Check sheet for the modelled part. Datum: model origin and axes. Units: mm. A direction names the side the tool comes from. Give positions to 0.01 mm unless a question says otherwise; leave off trailing zeros. Write each loop counter-clockwise with the first axis right and the second up, starting at its lowest first coordinate (ties: lowest second). Pieces come first, ordered by that corner, then holes. Notation, with made-up numbers: M 12.5,16 L 45.5,16 A20 cw 45.5,50 Z; hole C 61.5,77 d3. An arc over 180 degrees is marked long. Write item = value, one per line. Start each with the question number.
1) Sectioned sample at C-C, the plane x = 1. Record the cut outline in (y, z).
2) Sectioned sample at A-A, the plane y = -17.25. Record the cut outline in (x, z) (3 decimals), then the cut area to 3 significant figures.
3) Draft check along X on faces 1 (the face through (12.7, -3, 5)), 2 (the face through (19.297, -13.993, 1.565)), 3 (the face through (16, -11, 3.175)). Enter one of: pulls with the +X half, pulls with the -X half, needs draft (parallel to the pull), parting line crosses it, or undercut.
4) Sectioned sample at B-B, the plane z = 1. Record the cut outline in (x, y) (3 decimals), then the cut area to 3 significant figures.
5) Sectioned sample at D-D, the plane x = 19.05. Record the cut outline in (y, z) (3 decimals).
6) Scan lines: L1, parallel to X at y = -16.5, z = 3; L2, parallel to X at y = -3.25, z = 5.5; L3, parallel to X at y = -3, z = 0.5. Record each from-to range of solid material in increasing order.
7) Set-up check for faces 4 (the face through (-12.7, -3, 5)), 5 (the face through (0, -12.7, 3)), 6 (the face through (-9.935, -11.591, 3.836)): record each of +Z, -Z, +X, -X, +Y, -Y from which the full face is reachable in a straight line by a thin tool's end or side.
8) Gauge pin test, flat ends, axial feed: pin 1 (2 mm diameter, centred on y = -7.5, z = 10, fed in from +X); pin 2 (3 mm diameter, centred on x = -6, y = -11, fed in from +Z); pin 3 (5 mm diameter, centred on x = 14.5, y = -8, fed in from +Z). Record the tip position at first contact, or that the pin passes through.
from build123d import *

# Parameters (mm, degrees)
BOSS_EXTRUDE1_DEPTH   = 12.7
BOSS_EXTRUDE2_DEPTH   = 3.175
FILLET1_R             = 6.35
F_6_CLEARANCE_HOLE1_D = 3.7973


with BuildPart() as part:
    # Sketch1 → Boss-Extrude1 (new body)
    with BuildSketch(Plane.XY):
        with BuildLine():
            Line((-12.7, 0), (12.7, 0))
            Line((12.7, 0), (12.7, -6.35))
            ThreePointArc((12.7, -6.35), (10.840128061, -10.840128061), (6.35, -12.7))
            Line((6.35, -12.7), (-6.35, -12.7))
            ThreePointArc((-6.35, -12.7), (-10.840128061, -10.840128061), (-12.7, -6.35))
            Line((-12.7, -6.35), (-12.7, 0))
        make_face()
    extrude(amount=BOSS_EXTRUDE1_DEPTH)

    # Sketch2 → Boss-Extrude2 (add)
    with BuildSketch(Plane(origin=(0, 0, 0), x_dir=(-1, 0, 0), z_dir=(0, 0, -1))):
        with BuildLine():
            Line((12.7, 0), (12.7, -6.35))
            ThreePointArc((12.7, -6.35), (11.795080078, -9.617048047), (9.338235294, -11.952941176))
            Line((9.338235294, -11.952941176), (20.544117647, -5.976470588))
            ThreePointArc((20.544117647, -5.976470588), (22.130202438, -2.404949391), (19.05, 0))
            Line((19.05, 0), (12.7, 0))
        make_face()
        with BuildLine():
            Line((-12.7, 0), (-21.727676004, -14.168929598))
            ThreePointArc((-21.727676004, -14.168929598), (-20.856846986, -18.485733416), (-16.51, -17.78))
            ThreePointArc((-16.51, -17.78), (-12.029612663, -14.040774674), (-6.35, -12.7))
            ThreePointArc((-6.35, -12.7), (-10.840128061, -10.840128061), (-12.7, -6.35))
            Line((-12.7, -6.35), (-12.7, 0))
        make_face()
    extrude(amount=-BOSS_EXTRUDE2_DEPTH)

    # Fillet1
    fillet1_edges = [part.edges().sort_by_distance(p)[0] for p in [
        (-12.7, -3.175, 12.7),
        (-10.840128061, -10.840128061, 12.7),
        (0, -12.7, 12.7),
        (10.840128061, -10.840128061, 12.7),
        (12.7, -3.175, 12.7),
    ]]
    fillet(fillet1_edges, radius=FILLET1_R)

    # #6 Clearance Hole1 (through all)
    with Locations(Plane.XY.offset(3.175)):
        with Locations((-19.05, -3.175), (19.05, -15.875)):
            Hole(F_6_CLEARANCE_HOLE1_D / 2)


solid = part.part
Data:
q1.outline = M -12.7,0 L 0,0 L 0,12.7 L -6.35,12.7 A6.35 ccw -12.7,6.35 Z
q2.outline = M 16.09,0 L 17.741,0 L 17.741,3.175 L 16.09,3.175 Z; M 20.359,0 L 21.912,0 L 21.912,3.175 L 20.359,3.175 Z
q2.area = 10.2 mm2
q3.face_1 = pulls with the +X half
q3.face_2 = undercut
q3.face_3 = needs draft
q4.outline = M -20.544,-5.976 L -9.338,-11.953 A6.35 ccw -6.35,-12.7 L 6.35,-12.7 A12.7 cw 16.51,-17.78 A3.175 ccw 21.728,-14.169 L 12.7,0 L -19.05,0 A3.175 ccw Z; hole C -19.05,-3.175 d3.797; hole C 19.05,-15.875 d3.797
q4.area = 462 mm2
q5.outline = M -19.05,0 L -17.774,0 L -17.774,3.175 L -19.05,3.175 Z; M -13.976,0 L -9.966,0 L -9.966,3.175 L -13.976,3.175 Z
q6.L1 = 15.41 to 17.26, 20.84 to 22.16
q6.L2 = -12.7 to 12.7
q6.L3 = -22.22 to -20.94, -17.16 to 14.61
q7.face_4 = +Z, -X, +Y, -Y
q7.face_5 = +Z, -Z, -X, -Y
q7.face_6 = +Z, -X, -Y
q8.pin_1 = 12.04
q8.pin_2 = 11.86
q8.pin_3 = 8.9
